Can you work these out from the model? Positions are in its coordinate system, mm. A direction names the side the tool comes from. Give positions to 0.01 mm unless a question says otherwise; leave off trailing zeros. Order: outer loops, then holes, each group sorted by start corner. A loop starts at its lowest first (then second) coordinate and runs counter-clockwise, first axis right, second up.
Item 1: I want a section at B-B, the plane z = 7. Write out the boundary of the cut face in (x, y).
Item 2: Which directions (+Z, -Z, +X, -X, +Y, -Y) give clear straight access to the entire face, cutting with the end or side of a thin tool? Please do faces 4 (the cylindrical face through (108.076, -6.876, 12.818)), 5 (the flat face through (-9.165, 6, 15)), 6 (the flat face through (113.665, 5, 15)), 7 (the cylindrical face through (106, 10, 15)).
Item 3: I want a section at D-D, the plane z = 15. Write out the boundary of the cut face in (x, y), then the cut area to 3 significant figures.
Item 4: If I drill on line 1 along X through (y, z) = (-0.5, 20); line 2 along Y through (x, z) = (104.5, 28.4); line 3 along X through (y, z) = (-5.5, 28), over which ranges is the centre line in solid material (lowest first)?
Item 5: I'm going to push flat-ended pins straight in: pin 1 Ø7.5 at (x, y) = (48.5, -7) entering from -Z; pin 2 Ø2 at (y, z) = (9, 10.5) entering from -X; pin 3 Ø3 at (x, z) = (86.5, 23) entering from -Y. Where does each tip first touch, or does it pass through?
Item 6: I want a section at A-A, the plane x = 52.25. Write out the boundary of the cut face in (y, z).
Item 7: If we mould it in two halves opening along Z, with no side actions, what happens to faces 1 (the flat face through (50, -5, 25)), 2 (the flat face through (51, 6, 30)), 3 (the cylindrical face through (0.07, 9.83, 13.5))? For each: +Z half, -Z half, draft (parallel to the pull), parting line (faces both ways), or undercut.
Item 8: I want a section at C-C, the plane y = 0. Count the separate pieces of the cut face and the enclosed holes in it, then the cut area to 4 significant figures.
```python
from build123d import *

# Parameters (mm, degrees)
SKETCH1_R           = 5.25
SKETCH1_R_2         = 7.75
SKETCH1_R_3         = 1.75
BOSS_EXTRUDE2_DEPTH = 30
FILLET5_R           = 5
BOSS_EXTRUDE3_START = -4
SKETCH2_R           = 7.75
SKETCH2_R_2         = 6
BOSS_EXTRUDE3_DEPTH = 4
CUT_EXTRUDE1_REACH  = 122.579
SKETCH3_R           = 1.5
CUT_EXTRUDE3_DEPTH  = 25


with BuildPart() as part:
    # Sketch1 → Boss-Extrude2 (new body)
    with BuildSketch(Plane.XY):
        with BuildLine():
            ThreePointArc((-9.16515139, 4), (0, -10), (9.16515139, 4))
            Line((9.16515139, 4), (42.003049234, 4))
            ThreePointArc((42.003049234, 4), (52.25, -11), (62.496950766, 4))
            Line((62.496950766, 4), (95.33484861, 4))
            ThreePointArc((95.33484861, 4), (104.5, -10), (113.66515139, 4))
            Line((113.66515139, 4), (113.66515139, 12))
            Line((113.66515139, 12), (-9.16515139, 12))
            Line((-9.16515139, 12), (-9.16515139, 4))
        make_face()
        with Locations((52.25, 0)):
            Circle(SKETCH1_R, mode=Mode.SUBTRACT)
        Circle(SKETCH1_R_2, mode=Mode.SUBTRACT)
        with Locations((60.25, 0)):
            Circle(SKETCH1_R_3, mode=Mode.SUBTRACT)
        with Locations((44.25, 0)):
            Circle(SKETCH1_R_3, mode=Mode.SUBTRACT)
        with Locations((104.5, 0)):
            Circle(SKETCH1_R_2, mode=Mode.SUBTRACT)
    extrude(amount=BOSS_EXTRUDE2_DEPTH)

    # Fillet5
    fillet5_edges = [part.edges().sort_by_distance(p)[0] for p in [
        (-9.16515139, 12, 15),
        (113.66515139, 12, 15),
    ]]
    fillet(fillet5_edges, radius=FILLET5_R)

    # Sketch2 → Boss-Extrude3 (add)
    # profile 1 of 2: a face of its own
    with BuildSketch(Plane.XY.offset(30).offset(BOSS_EXTRUDE3_START)):
        Circle(SKETCH2_R)
        Circle(SKETCH2_R_2, mode=Mode.SUBTRACT)
    # profile 2 of 2: a face of its own
    with BuildSketch(Plane.XY.offset(30).offset(BOSS_EXTRUDE3_START)):
        with Locations((104.5, 0)):
            Circle(SKETCH2_R)
        with Locations((104.5, 0)):
            Circle(SKETCH2_R_2, mode=Mode.SUBTRACT)
    extrude(amount=BOSS_EXTRUDE3_DEPTH)

    # Sketch3 → Cut-Extrude1 (cut, up to next)
    with BuildSketch(Plane(origin=(0, 12, 0), x_dir=(1, 0, 0), z_dir=(0, 1, 0)), mode=Mode.PRIVATE) as cut_extrude1_sk1:
        with Locations(Location((0, -15, 0), (0, 0, 270))):
            Circle(SKETCH3_R)
    cut_extrude1_tool1 = extrude(cut_extrude1_sk1.sketch, amount=-CUT_EXTRUDE1_REACH, mode=Mode.PRIVATE) & part.part
    # Sketch3 → Cut-Extrude1 (cut, up to next)
    with BuildSketch(Plane(origin=(0, 12, 0), x_dir=(1, 0, 0), z_dir=(0, 1, 0)), mode=Mode.PRIVATE) as cut_extrude1_sk2:
        with Locations(Location((104.5, -15, 0), (0, 0, 270))):
            Circle(SKETCH3_R)
    cut_extrude1_tool2 = extrude(cut_extrude1_sk2.sketch, amount=-CUT_EXTRUDE1_REACH, mode=Mode.PRIVATE) & part.part
    add(cut_extrude1_tool1.solids().sort_by_distance((0, 12, 15))[0], mode=Mode.SUBTRACT)
    add(cut_extrude1_tool2.solids().sort_by_distance((104.5, 12, 15))[0], mode=Mode.SUBTRACT)

    # Sketch5 → Cut-Extrude3 (cut)
    with BuildSketch(Plane(origin=(0, 0, 0), x_dir=(-1, 0, 0), z_dir=(0, 0, -1))):
        with BuildLine():
            Line((-62.496950766, 4), (-42.003049234, 4))
            ThreePointArc((-42.003049234, 4), (-52.25, -11), (-62.496950766, 4))
        make_face()
    extrude(amount=-CUT_EXTRUDE3_DEPTH, mode=Mode.SUBTRACT)


solid = part.part
```
Results list:
1. outline: (-9.17, 4) arc R10 ccw (long way) to (9.17, 4) - (48.85, 4) arc R5.25 cw to (55.65, 4) - (95.33, 4) arc R10 ccw (long way) to (113.67, 4) - (113.67, 7) arc R5 ccw to (108.67, 12) - (-4.17, 12) arc R5 ccw to (-9.17, 7) - close; hole circle Ø15.5 at (0, 0); hole circle Ø15.5 at (104.5, 0)
2. face 4: -Z
2. face 5: +Z, -Z, -X, +Y
2. face 6: +Z, -Z, +X, +Y
2. face 7: +Y
3. outline: (-9.17, 4) arc R10 ccw (long way) to (9.17, 4) - (48.85, 4) arc R5.25 cw to (55.65, 4) - (95.33, 4) arc R10 ccw (long way) to (113.67, 4) - (113.67, 7) arc R5 ccw to (108.67, 12) - (106, 12) - (106, 7.6) arc R7.75 cw (long way) to (103, 7.6) - (103, 12) - (1.5, 12) - (1.5, 7.6) arc R7.75 cw (long way) to (-1.5, 7.6) - (-1.5, 12) - (-4.17, 12) arc R5 ccw to (-9.17, 7) - close
3. area: 1,030 mm2
4. line 1: x = -9.99 to -7.73, 7.73 to 9.99, 94.51 to 96.77, 112.23 to 114.49
4. line 2: y = -10 to -6, 6 to 12
4. line 3: x = -8.35 to -2.4, 2.4 to 8.35, 42.72 to 61.78, 96.15 to 102.1, 106.9 to 112.85
5. pin 1: stops at z = 25
5. pin 2: stops at x = -9.06
5. pin 3: stops at y = 4
6. outline: (-11, 25) - (-5.25, 25) - (-5.25, 30) - (-11, 30) - close; (5.25, 0) - (12, 0) - (12, 30) - (5.25, 30) - close
7. face 1: -Z half
7. face 2: +Z half
7. face 3: undercut
8. separate pieces: 8
8. enclosed holes: 0
8. area: 320.5 mm2
